Source: CAD feature listing. Evaluate the final solid. Frame: model axes, mm. A direction names the side the tool comes from. Give positions to 0.01 mm unless a question says otherwise; leave off trailing zeros. Loops run counter-clockwise (first coordinate to the right, second up) from the corner with the lowest first, then second, coordinate; pieces in that order, holes last.
```python
from build123d import *

# Parameters (mm, degrees)
F1_DEPTH = 3.5
F0_W     = 29.5
F0_H     = 29.5
F2_DEPTH = 1
F3_SIZE  = 1
F5_DEPTH = 2.5
F6_W     = 1
F6_H     = 5
F6_W_2   = 6
F6_H_2   = 1
F7_DEPTH = 1.5
F8_DEPTH = 0.5


with BuildPart() as f1:
    # F0 (on Top) → F1 (new body)
    with BuildSketch(Plane.XY):
        Polygon((12.8, -12.8), (12.8, 12.8), (-12.8, 12.8), (-12.8, 0.95), (-8.65, 0.95), (-8.55, 0.95), (-8.55, -9.05), (-8.65, -9.05), (-12.8, -9.05), (-12.8, -12.8), align=None)
        Polygon((2.55, -7.55), (8.95, -7.55), (8.95, -12.2), (2.55, -12.2), (2.55, -7.642402336), align=None, mode=Mode.SUBTRACT)
    extrude(amount=F1_DEPTH)

    # F0 (on Top) → F2 (join)
    with BuildSketch(Plane.XY):
        Rectangle(F0_W, F0_H)
        Polygon((-12.8, 12.8), (12.8, 12.8), (12.8, -12.8), (-12.8, -12.8), (-12.8, -9.05), (-12.8, 0.95), align=None, mode=Mode.SUBTRACT)
    extrude(amount=F2_DEPTH)

    # F3
    f3_edges = [f1.edges().sort_by_distance(p)[0] for p in [
        (14.75, 14.75, 0.5),
        (14.75, -14.75, 0.5),
        (-14.75, -14.75, 0.5),
        (-14.75, 14.75, 0.5),
    ]]
    chamfer(f3_edges, length=F3_SIZE)

    # F4 (on face) → F5 (cut)
    with BuildSketch(Plane.XY.offset(3.5)):
        Polygon((11, -11), (11, 11), (-11, 11), (-11, 0.95), (-8.55, 0.95), (-8.55, -9.05), (-11, -9.05), (-11, -11), (2.55, -11), (2.55, -7.55), (8.95, -7.55), (8.95, -11), align=None)
    extrude(amount=-F5_DEPTH, mode=Mode.SUBTRACT)

    # F6 (on face) → F7 (cut)
    with BuildSketch(Plane.XY.offset(3.5)):
        with Locations((11.5, -5.8585465327)):
            Rectangle(F6_W, F6_H)
        with Locations((-5.983454667, -11.5)):
            Rectangle(F6_W_2, F6_H_2)
    extrude(amount=-F7_DEPTH, mode=Mode.SUBTRACT)

    # F8 (cut): a face of the model
    f8_faces = [f1.faces().sort_by_distance(p)[0] for p in [
        (-12.437961328, -10.925, 3.5),
    ]]
    extrude(f8_faces, amount=-F8_DEPTH, mode=Mode.SUBTRACT)


solid = f1.part
```
(1) First-contact query: pin 1 (0.5 mm diameter, centred on x = 11.5, y = -5.5, fed in from +Z); pin 2 (0.6 mm diameter, centred on x = -3.5, z = 2, fed in from +Y); pin 3 (1.5 mm diameter, centred on x = -10.5, z = 2, fed in from -Y). Flat tips, straight axial feed; report the tip coordinate or a pass-through.
A:
pin 1: stops at z = 2
pin 2: stops at y = 12.8
pin 3: stops at y = -12.8
(2) Section D-D, the plane x = -0.5. Return the cut outline in (y, z), then the cut area to 3 significant figures.
A:
outline: (-14.75, 0) - (14.75, 0) - (14.75, 1) - (12.8, 1) - (12.8, 3) - (11, 3) - (11, 1) - (-11, 1) - (-11, 3) - (-12.8, 3) - (-12.8, 1) - (-14.75, 1) - close
area: 36.7 mm2
(3) Mould query, pull axis X, two halves, no side actions, for faces 5 (the flat face through (0, 0, 1)), 6 (the flat face through (11.5, -5.8, 2)), 7 (the flat face through (-12.8, 7, 2)), 8 (the flat face through (6, -12.2, 1)). Classes: pulls with the +X half, pulls with the -X half, needs draft (parallel to the pull), parting line crosses it, or undercut.
A:
face 5: undercut
face 6: needs draft
face 7: pulls with the -X half
face 8: undercut
(4) Reachability of faces 1 (the flat face through (-8.55, -4, 0.5)), 2 (the flat face through (-2.983, -11.5, 2.5)), 3 (the flat face through (-12.8, -11, 2)), 4 (the flat face through (12, -5.9, 2.5)) from +Z, -Z, +X, -X, +Y, -Y: full face, straight path, thin tool, end or side. Return the list, or none.
A:
face 1: +Z, -Z
face 2: +Z
face 3: +Z, -X, +Y, -Y
face 4: +Z, -X
(5) Section C-C, the plane z = 0.6. Return the cut outline in (x, y).
A:
outline: (-14.75, -13.75) - (-13.75, -14.75) - (13.75, -14.75) - (14.75, -13.75) - (14.75, 13.75) - (13.75, 14.75) - (-13.75, 14.75) - (-14.75, 13.75) - close; hole (-12.8, -9.05) - (-8.55, -9.05) - (-8.55, 0.95) - (-12.8, 0.95) - close; hole (2.55, -12.2) - (8.95, -12.2) - (8.95, -7.55) - (2.55, -7.55) - close
(6) Section A-A, the plane x = -10.5. Return the cut outline in (y, z).
A:
outline: (-14.75, 0) - (-9.05, 0) - (-9.05, 1) - (-11, 1) - (-11, 3) - (-12.8, 3) - (-12.8, 1) - (-14.75, 1) - close; (0.95, 0) - (14.75, 0) - (14.75, 1) - (12.8, 1) - (12.8, 3) - (11, 3) - (11, 1) - (0.95, 1) - close
(7) Section B-B, the plane y = -5. Return the cut outline in (x, z), then the cut area to 4 significant figures.
A:
outline: (-14.75, 0) - (-12.8, 0) - (-12.8, 1) - (-14.75, 1) - close; (-8.55, 0) - (14.75, 0) - (14.75, 1) - (12.8, 1) - (12.8, 3) - (12, 3) - (12, 2) - (11, 2) - (11, 1) - (-8.55, 1) - close
area: 27.85 mm2
(8) Ray query, line 1 along X through (y, z) = (-8.5, 0.85); line 2 along Y through (x, z) = (1.25, 1.1); line 3 along Y through (x, z) = (-12.5, 0.8). Return the intervals inside material, ascending.
A:
line 1: x = -14.75 to -12.8, -8.55 to 2.55, 8.95 to 14.75
line 2: y = -12.8 to -11, 11 to 12.8
line 3: y = -14.75 to -9.05, 0.95 to 14.75
